Source: CAD feature listing. Evaluate the final solid. Frame: model axes, mm. Give positions to 0.01 mm unless a question says otherwise; leave off trailing zeros. Write each loop counter-clockwise with the first axis right and the second up, starting at its lowest first coordinate (ties: lowest second). Pieces come first, ordered by that corner, then holes. Notation, with made-up numbers: M 47,-7.5 L 57,-7.5 A38 cw 57,31.5 Z; hole C 85.25,-11 d9. An arc over 180 degrees is marked long. Use CSV: the item, a comma, the result in double quotes. Start each with the question number.
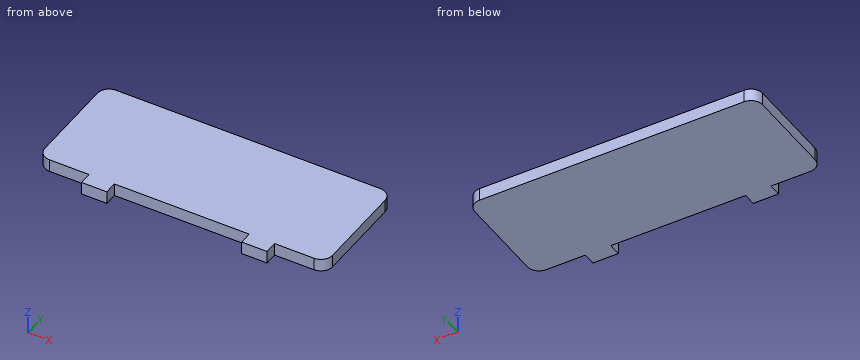
from build123d import *

# Parameters (mm, degrees)
BASE_FLANGE1_DEPTH = 2.3
SKETCH6_W          = 4.6
SKETCH6_H          = 2.3
TAB1_DEPTH         = 2.3


# Sheet-metal steps are written as plain solids
with BuildPart() as part:
    # Model → Base-Flange1 (new body)
    with BuildSketch(Plane.XY):
        with BuildLine():
            Line((286.92374396, -389.094251747), (238.923745329, -389.094251747))
            add(Edge.make_bspline(
                [(238.923745329, -389.094251747), (237.7557503, -389.094251747), (236.80552837, -390.044409082), (236.80552837, -391.212296452)],
                knots=[1, 1, 1, 1, 2, 2, 2, 2], degree=3))
            Line((236.80552837, -391.212296452), (236.80552837, -407.212353414))
            add(Edge.make_bspline(
                [(236.80552837, -407.212353414), (236.80552837, -408.380240783), (237.7557503, -409.330398118), (238.923745329, -409.330398118)],
                knots=[3, 3, 3, 3, 4, 4, 4, 4], degree=3))
            Line((238.923745329, -409.330398118), (286.92374396, -409.330398118))
            add(Edge.make_bspline(
                [(286.92374396, -409.330398118), (288.09163133, -409.330398118), (289.041788665, -408.380240783), (289.041788665, -407.212353414)],
                knots=[5, 5, 5, 5, 6, 6, 6, 6], degree=3))
            Line((289.041788665, -407.212353414), (289.041788665, -391.212296452))
            add(Edge.make_bspline(
                [(289.041788665, -391.212296452), (289.041788665, -390.044409082), (288.09163133, -389.094251747), (286.92374396, -389.094251747)],
                knots=[7, 7, 7, 7, 8, 8, 8, 8], degree=3))
        make_face()
    extrude(amount=-BASE_FLANGE1_DEPTH)

    # Sketch6 → Tab1 (add)
    with BuildSketch(Plane.XY):
        with Locations((248.373744645, -410.480398118)):
            Rectangle(SKETCH6_W, SKETCH6_H)
        with Locations((277.473744645, -410.480398118)):
            Rectangle(SKETCH6_W, SKETCH6_H)
    extrude(amount=-TAB1_DEPTH)


solid = part.part
Item 1: Material intervals for probe 1 along Y at (x, z) = (280.5, -1.7); probe 2 along X at (y, z) = (-407.5, -1.1), sorted ascending.
Item 2: Section A-A (x = 258). Return the cut outline in (y, z).
Item 3: Contact query for flat-ended pins moving along their axis: pin 1 Ø0.7 at (y, z) = (-411, -1) entering from -X; pin 2 Ø1.1 at (y, z) = (-410, -1) entering from +X; pin 3 Ø1.2 at (x, z) = (283.5, -0.5) entering from -Y. Output: stop coordinate, or through.
Output values:
1,probe 1,"y = -409.33 to -389.09"
1,probe 2,"x = 236.82 to 289.02"
2,outline,"M -409.33,-2.3 L -389.09,-2.3 L -389.09,0 L -409.33,0 Z"
3,pin 1,"stops at x = 246.07"
3,pin 2,"stops at x = 279.77"
3,pin 3,"stops at y = -409.33"
